Verification items for the finished model (mm, model axes). A direction names the side the tool comes from. Give positions to 0.01 mm unless a question says otherwise; leave off trailing zeros. Write each loop counter-clockwise with the first axis right and the second up, starting at its lowest first coordinate (ties: lowest second). Pieces come first, ordered by that corner, then holes. Notation, with made-up numbers: M -0.5,61 L 51.5,61 A20 ccw 51.5,84 Z; hole C -29.75,51 d3. An arc over 180 degrees is marked long. Write item = value, one per line.
from build123d import *

# Parameters (mm, degrees)
F0_R     = 63.4990492705
F1_DEPTH = 127
F1_TAPER = -20
F2_R     = 25.4
F3_SIZE  = 63.5
F4_T     = -12.7


# Not quite as in the source:
# - a shell that OpenCascade refuses in one call is made with other operations: the cavity is built on its own and cut out


with BuildPart() as f1:
    # F0 (on Front) → F1 (new body, symmetric)
    with BuildSketch(Plane.XZ):
        with Locations((1.6070879065, 0)):
            Circle(F0_R)
    extrude(amount=F1_DEPTH, both=True, taper=F1_TAPER)

    # F2
    f2_edges = [f1.edges().sort_by_distance(p)[0] for p in [
        (-108.116181, -127, 0),
    ]]
    fillet(f2_edges, radius=F2_R)

    # F3
    f3_edges = [f1.edges().sort_by_distance(p)[0] for p in [
        (-108.116181, 127, 0),
    ]]
    chamfer(f3_edges, length=F3_SIZE)

    # F4: a shell. OpenCascade refuses it in one call, so the cavity is built on its own and cut out:
    # the body offset inwards by the wall thickness, plus a prism from it out through each open face.
    f4_core = offset(f1.part, amount=F4_T, kind=Kind.INTERSECTION, mode=Mode.PRIVATE)
    f4_exits = [f4_core.faces().sort_by_distance(p)[0] for p in [
        (1.607088, -114.3, 0),
    ]]
    add(f4_core, mode=Mode.SUBTRACT)
    extrude(f4_exits, amount=-F4_T, mode=Mode.SUBTRACT)


solid = f1.part
1) Draft check along Z on faces 4 (the flat face through (1, 127, 1)), 5 (the conical face through (-7.34, 111.93, -40.29)), 6 (the conical face through (-13.081, 11.693, -66.144)). Enter one of: +Z half, -Z half, draft (parallel to the pull), parting line (faces both ways), or undercut.
From the geometry:
face_4 = draft
face_5 = undercut
face_6 = parting line
2) Tool access check on faces 1 (the conical face through (-11.41, -27.7, -58.64)), 2 (the flat face through (1, 114.3, 1)), 3 (the conical face through (47.631, 124.103, 14.494)). Record the directions out of +Z, -Z, +X, -X, +Y, -Y that give a thin tool (end or side, any length) a straight path to the whole face; none if there is none.
From the geometry:
face_1 = none
face_2 = -Y
face_3 = +Y
3) Cross-section at A-A on y = 108.5. Record the boundary of the cut face in (x, z).
From the geometry:
outline = C 1.61,0 d118.35; hole C 1.61,0 d87.35
4) Depth check by flat-ended pin: P1, Ø1, axis at x = -11.5, z = -34, coming from the -Y side; P2, Ø6, axis at x = 6, y = 38.5, coming from the -Z side; P3, Ø2, axis at y = 38, z = 0.5, coming from the -X side. Enter the tip coordinate at first touch or a pass-through.
From the geometry:
P1 = 114.3
P2 = -78.49
P3 = -76.09
5) Cross-section at C-C on y = -23.5. Record the boundary of the cut face in (x, z).
From the geometry:
outline = C 1.61,0 d144.1; hole C 1.61,0 d117.07
6) Cross-section at B-B on x = -66. Count the separate pieces of the cut face and the enclosed holes in it, plus the area to 3 significant figures.
From the geometry:
separate_pieces = 2
enclosed_holes = 1
area = 11,300 mm^2
7) Material ranges on probe 1 along Y at (x, z) = (-55, 58.5); probe 2 along X at (y, z) = (-124, 0); probe 3 along X at (y, z) = (-93, -66), recorded low to high. Write a range as from..to.
From the geometry:
probe_1 = -125.72..-111.5, -86.33..-49.19, 49.19..76.76
probe_2 = -83.82..-71.84, 75.06..87.03
probe_3 = -69.95..-50.08, 53.3..73.17
